from build123d import *

# Parameters (mm, degrees)
F0_W     = 2
F0_H     = 2
F0_W_2   = 11
F0_H_2   = 28
F0_W_3   = 35
F1_DEPTH = 60
F2_R     = 10


with BuildPart() as f1:
    # F0 (on Front) → F1 (new body)
    with BuildSketch(Plane.XZ):
        with Locations((1, 1)):
            Rectangle(F0_W, F0_H)
        with Locations((7.5, 1)):
            Rectangle(F0_W_2, F0_H)
        with Locations((1, 16)):
            Rectangle(F0_W, F0_H_2)
        with Locations((14, 1)):
            Rectangle(F0_W, F0_H)
        with Locations((32.5, 1)):
            Rectangle(F0_W_3, F0_H)
        with Locations((14, 16)):
            Rectangle(F0_W, F0_H_2)
    extrude(amount=F1_DEPTH)

    # F2
    f2_edges = [f1.edges().sort_by_distance(p)[0] for p in [
        (14, -60, 30),
        (1, -60, 30),
        (14, 0, 30),
        (1, 0, 30),
        (15, -30, 2),
        (50, 0, 1),
        (50, -60, 1),
    ]]
    fillet(f2_edges, radius=F2_R)


solid = f1.part
Geometry check sheet. Reference: the model listing, model coordinates, mm. A direction names the side the tool comes from. Coordinates: 2 decimals unless noted, no trailing zeros. Order: outer loops, then holes, each group sorted by start corner. A loop starts at its lowest first (then second) coordinate and runs counter-clockwise, first axis right, second up. Notation, with made-up numbers: (-24, 29.25) - (28, 29.25) arc R17 cw to (28, 60.25) - close; hole circle Ø3 at (24.5, 19). An arc over 180 degrees is marked (long way). One line per item, written item: value.
(1) Sectioned sample at C-C (z = 4). Enter the section's corners in (x, y).
Data:
outline: (0, -60) - (2, -60) - (2, 0) - (0, 0) - close; (13, -60) - (19, -60) - (19, 0) - (13, 0) - close
(2) Depth check by flat-ended pin: pin 1 Ø9 at (y, z) = (-41, 18) entering from +X; pin 2 Ø7.5 at (x, y) = (40, -27) entering from +Z; pin 3 Ø5 at (x, y) = (21, -18) entering from +Z. Enter the tip coordinate at first touch or a pass-through.
Data:
pin 1: stops at x = 15
pin 2: stops at z = 2
pin 3: stops at z = 4.4
(3) Thickness scan on probe 1 along X at (y, z) = (-46, 27.5); probe 2 along X at (y, z) = (-29, 10); probe 3 along Z at (x, y) = (34.5, -36). Record the ranges inside material, lowest first. Write a range as from..to.
Data:
probe 1: x = 0..2, 13..15
probe 2: x = 0..2, 13..15.2
probe 3: z = 0..2
(4) Access from +Z, -Z, +X, -X, +Y, -Y to the whole of each face (thin tool, end or side, straight path). Record for faces 1 (the face through (8, -30, 2)), 2 (the face through (15, -30, 21)), 3 (the face through (14, -30, 30)).
Data:
face 1: +Z, +Y, -Y
face 2: +Z, +X, +Y, -Y
face 3: +Z, +X, -X, +Y, -Y
(5) Sectioned sample at B-B (y = -41). Enter the section's corners in (x, z), and give its area (3 significant figures).
Data:
outline: (0, 0) - (50, 0) - (50, 2) - (25, 2) arc R10 cw to (15, 12) - (15, 30) - (13, 30) - (13, 2) - (2, 2) - (2, 30) - (0, 30) - close
area: 233 mm^2
(6) Sectioned sample at A-A (z = 19). Enter the section's corners in (x, y), and give its area (3 significant figures).
Data:
outline: (0, -60) - (2, -60) - (2, 0) - (0, 0) - close; (13, -60) - (15, -60) - (15, 0) - (13, 0) - close
area: 240 mm^2
(7) Release check for a two-part mould opening along X. For faces 4 (the face through (38, -30, 2)), 5 (the face through (2, -30, 16)), 6 (the face through (13, -30, 16)), 7 (the face through (50, -30, 1)) record: +X half, -X half, draft (parallel to the pull), parting line (faces both ways), or undercut.
Data:
face 4: draft
face 5: undercut
face 6: undercut
face 7: +X half
(8) Sectioned sample at D-D (x = 34.5). Enter the section's corners in (y, z), and give its area (3 significant figures).
Data:
outline: (-60, 0) - (0, 0) - (0, 2) - (-60, 2) - close
area: 120 mm^2
